Build history of the part. All positions in model axes, mm. A direction names the side the tool comes from. Round coordinates to 2 decimals unless told otherwise and drop trailing zeros. Order: outer loops, then holes, each group sorted by start corner. A loop starts at its lowest first (then second) coordinate and runs counter-clockwise, first axis right, second up. Notation, with made-up numbers: (32, 64) -> (63, 64) arc R20 cw to (63, 94) -> close; hole circle Ø2 at (54, 54). An arc over 180 degrees is marked (long way). Write item = value, one per line.
from build123d import *

# Parameters (mm, degrees)
F0_W          = 21
F0_H          = 20
F0_W_2        = 19
F0_H_2        = 18
F0_W_3        = 18
F0_H_3        = 17
F0_W_4        = 11.5
F0_H_4        = 11.5
F1_DEPTH      = 1
F2_W          = 21
F2_H          = 20
F2_W_2        = 19
F2_H_2        = 18
F3_DEPTH      = 7
F4_W          = 19
F4_H          = 18
F4_W_2        = 5
F4_H_2        = 5
F5_DEPTH      = 1
F5_DEPTH_BACK = 2
F7_D          = 2
F8_W          = 6
F8_H          = 6
F9_DEPTH      = 3
F10_W         = 6
F10_H         = 6
F11_DEPTH     = 3
F13_D         = 2


with BuildPart() as f1:
    # F0 (on Front) → F1 (new body)
    with BuildSketch(Plane.XZ):
        Rectangle(F0_W, F0_H)
        Rectangle(F0_W_2, F0_H_2, mode=Mode.SUBTRACT)
        Rectangle(F0_W_2, F0_H_2)
        Rectangle(F0_W_3, F0_H_3, mode=Mode.SUBTRACT)
        Rectangle(F0_W_3, F0_H_3)
        Rectangle(F0_W_4, F0_H_4, mode=Mode.SUBTRACT)
    extrude(amount=F1_DEPTH)

    # F2 (on face) → F3 (join)
    with BuildSketch(Plane.XZ.offset(1)):
        Rectangle(F2_W, F2_H)
        Rectangle(F2_W_2, F2_H_2, mode=Mode.SUBTRACT)
    extrude(amount=F3_DEPTH)

    # F4 (on face) → F5 (join, two sides)
    with BuildSketch(Plane.XZ.offset(8)) as f5_sk:
        Polygon((10.5, 2.5), (10.5, 10), (-10.5, 10), (-10.5, 2.5), (-10.5, -2.5), (-10.5, -10), (10.5, -10), (10.5, -2.5), align=None)
        Rectangle(F4_W, F4_H, mode=Mode.SUBTRACT)
        with Locations((13, 0)):
            Rectangle(F4_W_2, F4_H_2)
        with Locations((-13, 0)):
            Rectangle(F4_W_2, F4_H_2)
    extrude(amount=F5_DEPTH)
    extrude(f5_sk.sketch, amount=-F5_DEPTH_BACK)

    # F7 (through all)
    with Locations(Plane.XZ.offset(9)):
        with Locations((-12, 0), (12, 0)):
            Hole(F7_D / 2)

    # F8 (on face) → F9 (join)
    with BuildSketch(Plane(origin=(-10.5, 0, 0), x_dir=(0, -1, 0), z_dir=(-1, 0, 0))):
        with Locations((6, -7)):
            Rectangle(F8_W, F8_H)
    extrude(amount=F9_DEPTH)

    # F10 (on face) → F11 (join)
    with BuildSketch(Plane.YZ.offset(10.5)):
        with Locations((-6, -7)):
            Rectangle(F10_W, F10_H)
    extrude(amount=F11_DEPTH)

    # F13 (through all)
    with Locations(Plane(origin=(-13.5, 0, 0), x_dir=(0, -1, 0), z_dir=(-1, 0, 0))):
        with Locations((6, -7)):
            Hole(F13_D / 2)


solid = f1.part
Q1. Cut at D-D, the plane z = -7. List the corners of the cut face in (x, y), and give its area (3 significant figures).
Check values:
outline = (-13.5, -9) -> (-9.5, -9) -> (-9.5, -7) -> (-13.5, -7) -> close; (-13.5, -5) -> (-9.5, -5) -> (-9.5, -1) -> (9.5, -1) -> (9.5, -5) -> (13.5, -5) -> (13.5, -3) -> (10.5, -3) -> (10.5, 0) -> (-10.5, 0) -> (-10.5, -3) -> (-13.5, -3) -> close; (9.5, -9) -> (13.5, -9) -> (13.5, -7) -> (9.5, -7) -> close
area = 57.0 mm²
Q2. Cut at C-C, the plane y = -3.5. List the corners of the cut face in (x, z), and give its area (3 significant figures).
Check values:
outline = (-13.5, -10) -> (13.5, -10) -> (13.5, -4) -> (10.5, -4) -> (10.5, 10) -> (-10.5, 10) -> (-10.5, -4) -> (-13.5, -4) -> close; hole (-9.5, -9) -> (9.5, -9) -> (9.5, 9) -> (-9.5, 9) -> close
area = 114 mm²
Q3. Probe probe 1 along X at (y, z) = (-7.75, -4.75); probe 2 along Z at (x, y) = (3.5, -1.5); probe 3 along X at (y, z) = (-1.75, -7.5). List the from-to ranges inside material, lowest first.
Check values:
probe_1 = -13.5 to -9.5, 9.5 to 13.5
probe_2 = -10 to -9, 9 to 10
probe_3 = -10.5 to -9.5, 9.5 to 10.5
Q4. Cut at A-A, the plane x = 12. List the corners of the cut face in (y, z), and give its area (3 significant figures).
Check values:
outline = (-9, -10) -> (-3, -10) -> (-3, -4) -> (-9, -4) -> close; (-9, -2.5) -> (-6, -2.5) -> (-6, -1) -> (-9, -1) -> close; (-9, 1) -> (-6, 1) -> (-6, 2.5) -> (-9, 2.5) -> close; hole circle Ø2 at (-6, -7)
area = 41.9 mm²
Q5. Flat gauge pins, fed straight in: pin 1 (5.5 mm diameter, centred on x = -2, z = 1, fed in from -Y); pin 2 (3 mm diameter, centred on y = -5.5, z = -7.5, fed in from -X); pin 3 (2 mm diameter, centred on y = -7, z = 5.5, fed in from -X); pin 4 (0.9 mm diameter, centred on x = -11.5, y = -5, fed in from +Z). Where does each tip first touch, or does it go through?
Check values:
pin_1 = through
pin_2 = -13.5
pin_3 = -10.5
pin_4 = -4
Q6. Cut at B-B, the plane z = 4. List the corners of the cut face in (x, y), and give its area (3 significant figures).
Check values:
outline = (-10.5, -9) -> (-9.5, -9) -> (-9.5, -1) -> (-5.75, -1) -> (-5.75, 0) -> (-10.5, 0) -> close; (5.75, -1) -> (9.5, -1) -> (9.5, -9) -> (10.5, -9) -> (10.5, 0) -> (5.75, 0) -> close
area = 25.5 mm²
Q7. Which spindle directions (+Z, -Z, +X, -X, +Y, -Y) get a long thin tool onto all of the face, cutting with end or side? Do faces 4 (the face through (-0.1, -0.5, -5.75)), 5 (the face through (-13, -7, -2.5)), 6 (the face through (13, -7, -2.5)). Say none if no direction does.
Check values:
face_4 = +Y, -Y
face_5 = -X, +Y, -Y
face_6 = +X, +Y, -Y
Q8. Mould opens along X. For faces 1 (the face through (15.5, -8, 0)), 2 (the face through (-5.75, -0.5, -0.1)), 3 (the face through (-11.472, -6.737, -6.324)) say: released by +X, released by -X, zero draft, split by the parting line, or undercut.
Check values:
face_1 = released by +X
face_2 = undercut
face_3 = zero draft
